from build123d import *

# Parameters (mm, degrees)
F0_R     = 1.27
F1_DEPTH = 12.7


with BuildPart() as f1:
    # F0 (on Front) → F1 (new body)
    with BuildSketch(Plane.XZ):
        Polygon((0, 25.739086), (-22.112327, 12.70128), (-22.112327, -12.7), (0, -25.060914), (22.112327, -12.7), (22.112327, 12.70128), align=None)
        Polygon((-3.883768, -6.55597), (-3.92257, -18.866995), (-14.785223, -12.720766), align=None, mode=Mode.SUBTRACT)
        with Locations((0, -14.435457)):
            Circle(F0_R, mode=Mode.SUBTRACT)
        with Locations((-12.008663, -7.3025)):
            Circle(F0_R, mode=Mode.SUBTRACT)
        Polygon((-18.273105, 6.119124), (-7.619829, -0.05101), (-18.438062, -6.360705), align=None, mode=Mode.SUBTRACT)
        Polygon((-3.81, 0), (0, 3.81), (3.81, 0), (0, -3.81), align=None, mode=Mode.SUBTRACT)
        Polygon((3.883768, -6.55597), (14.785223, -12.720766), (3.92257, -18.866995), align=None, mode=Mode.SUBTRACT)
        with Locations((12.008663, -7.3025)):
            Circle(F0_R, mode=Mode.SUBTRACT)
        Polygon((18.273105, 6.119124), (18.438062, -6.360705), (7.619829, -0.05101), align=None, mode=Mode.SUBTRACT)
        with Locations((-12.008663, 7.30314)):
            Circle(F0_R, mode=Mode.SUBTRACT)
        Polygon((-14.492327, 12.70128), (-3.795361, 19.131543), (-3.795073, 6.607709), align=None, mode=Mode.SUBTRACT)
        with Locations((0, 14.774543)):
            Circle(F0_R, mode=Mode.SUBTRACT)
        Polygon((3.795073, 6.607709), (3.795361, 19.131543), (14.492327, 12.70128), align=None, mode=Mode.SUBTRACT)
        with Locations((12.008663, 7.30314)):
            Circle(F0_R, mode=Mode.SUBTRACT)
    extrude(amount=F1_DEPTH)


solid = f1.part
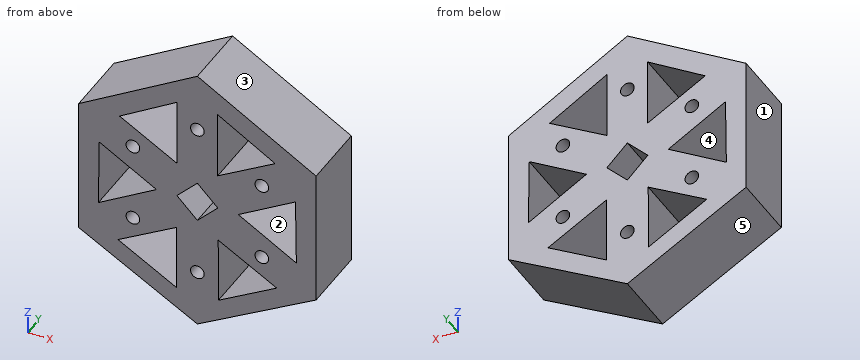
Source: CAD feature listing. Evaluate the final solid. Frame: model axes, mm. Face numbers are marked on the shaded views. A direction names the side the tool comes from. Give positions to 0.01 mm unless a question says otherwise; leave off trailing zeros. Write each loop counter-clockwise with the first axis right and the second up, starting at its lowest first coordinate (ties: lowest second). Pieces come first, ordered by that corner, then holes. Notation, with made-up numbers: M 18.25,75.25 L 45.25,75.25 A24 ccw 45.25,86.25 Z; hole C 21.5,28.5 d1. An arc over 180 degrees is marked long. Return JSON: item names as keys, results as strings. Group by question number.
1) Material intervals for line 1 along Z through (x, y) = (-14, -10.25); line 2 along X through (y, z) = (-2.25, -2); line 3 along Z through (x, y) = (-4.5, -3.25), sorted ascending. Write a range as [from, to].
2) Pin query (flat end, axial travel): P1, Ø2, axis at x = 15.5, y = -9.5, coming from the -Z side; P2, Ø2, axis at x = -2, z = -0.5, coming from the +Y side; P3, Ø4, axis at x = -14, y = -4.5, coming from the -Z side; P4, Ø6, axis at x = 9, y = -4.5, coming from the -Z side. Return the tip coordinate at first contact, or that it passes through.
3) Pull-direction query (Z, two-part tool) for the marked faces 3, 4 and 5; classes: pulls with the +Z half, pulls with the -Z half, needs draft (parallel to the pull), parting line crosses it, or undercut.
4) Cut plane C-C, the plane x = -2. Output: boundary loops of the cut face in (y, z), plus the area to 3 significant figures.
5) Cut plane B-B, the plane y = -7.75. Give the number of separate pieces and of enclosed holes in the cut face, plus the area to 3 significant figures.
6) Cut plane A-A, the plane x = -17. Output: boundary loops of the cut face in (y, z), plus the area to 3 significant figures.
7) Set-up query: the marked faces 1 and 2. Return all of +Z, -Z, +X, -X, +Y, -Y with unobstructed straight access to the full face (end or side cutting, diameter ignored); none if empty.
Recorded:
{
 "1": {"line 1": "z = [-17.23, -13.17], [-12.28, -3.77], [3.64, 12.42], [13, 17.48]", "line 2": "x = [-22.11, -18.38], [-10.96, -1.81], [1.81, 10.96], [18.38, 22.11]", "line 3": "z = [-22.55, -18.54], [-6.9, 7.01], [18.71, 23.09]"},
 "2": {"P1": "stops at z = -16.96", "P2": "stops at y = 0", "P3": "stops at z = -18.35", "P4": "stops at z = -21.71"},
 "3": {"face 3": "pulls with the +Z half", "face 4": "undercut", "face 5": "pulls with the -Z half"},
 "4": {"outline": "M -12.7,-23.94 L 0,-23.94 L 0,-1.81 L -12.7,-1.81 Z; M -12.7,1.81 L 0,1.81 L 0,24.56 L -12.7,24.56 Z", "area": "570 mm²"},
 "5": {"separate pieces": "1", "enclosed holes": "13", "area": "1,220 mm²"},
 "6": {"outline": "M -12.7,-15.56 L 0,-15.56 L 0,-5.52 L -12.7,-5.52 Z; M -12.7,5.38 L 0,5.38 L 0,15.72 L -12.7,15.72 Z", "area": "259 mm²"},
 "7": {"face 1": "+Z, -Z, -X, +Y, -Y", "face 2": "+Y, -Y"}
}
